Input: part model. Units: mm. Frame: model coordinates. A direction names the side the tool comes from. Coordinates: 2 decimals unless noted, no trailing zeros. Write each loop counter-clockwise with the first axis right and the second up, starting at its lowest first coordinate (ties: lowest second). Pieces come first, ordered by that corner, then holes. Notation, with made-up numbers: (-27.5, -12) - (17.5, -12) arc R35 ccw to (17.5, 22) - close; hole circle Ø4 at (8.25, 70). An arc over 180 degrees is marked (long way). One line per question, with ' | ' between items. Start each with the question number.
1) First-contact query: P1, Ø4, axis at x = -28, z = -2.5, coming from the +Y side; P2, Ø4, axis at x = -7.5, y = -10, coming from the +Z side. Flat tips, straight axial feed; report the tip coordinate or a pass-through.
2) Draft query along X for faces 1 (the flat face through (0, -6, 38.1)), 2 (the flat face through (-38.1, -10, 0)), 3 (the cylindrical face through (-24.984, -6.261, 18.408)). Return one class per face: released by +X, released by -X, zero draft, split by the parting line, or undercut.
3) Section query D-D on x = -28. Return loops of the section in (y, z), and give its area (3 significant figures).
4) Line query: line 1 (X direction, y = -5.5, z = 29.5); line 2 (Z direction, x = -29, y = -5.5); line 3 (Z direction, x = -25, y = -3.25). Output: solid intervals per line, ascending.
5) Section query C-C on y = -2.25. Give the number of separate pieces and of enclosed holes in the cut face, and give its area (3 significant figures).
6) Reachability of faces 4 (the flat face through (-29, -12.7, 29)), 5 (the cylindrical face through (35.927, -6.439, 35.809)), 6 (the flat face through (8, 0, 1)) from +Z, -Z, +X, -X, +Y, -Y: full face, straight path, thin tool, end or side. Return the list, or none.
7) Section query B-B on z = 0. Return loops of the section in (x, y) (3 decimals).
8) Section query A-A on x = 0. Return loops of the section in (y, z) (3 decimals), and give its area (4 significant figures).
```python
from build123d import *

# Parameters (mm, degrees)
F1_DEPTH = 12.7
F3_D     = 11.3284
F4_R     = 7.62
F5_W     = 76.2
F5_H     = 77.0487710834
F6_DEPTH = 7.62
F7_R     = 7.62


# Not quite as in the source:
# - a feature names something its author has since deleted; it is built from what else it names


with BuildPart() as f1:
    # F0 (on Front) → F1 (new body)
    with BuildSketch(Plane.XZ):
        Polygon((-38.1, -38.1), (38.1, -38.1), (38.1, -30.48), (38.1, 38.1), (-38.1, 38.1), align=None)
    extrude(amount=F1_DEPTH)

    # F3 (through all)
    with Locations(Plane.XZ.offset(12.7)):
        with Locations((-29.1592, 29.1592), (-14.5796, 29.1592), (0, 29.1592), (14.5796, 29.1592), (29.1592, 29.1592), (29.1592, 14.5796), (29.1592, 0), (29.1592, -14.5796), (29.1592, -29.1592), (14.5796, -29.1592), (14.5796, -14.5796), (14.5796, 0), (14.5796, 14.5796), (0, 14.5796), (0, 0), (0, -14.5796), (0, -29.1592), (-14.5796, -29.1592), (-14.5796, -14.5796), (-14.5796, 0), (-14.5796, 14.5796), (-29.1592, 14.5796), (-29.1592, 0), (-29.1592, -14.5796), (-29.1592, -29.1592)):
            Hole(F3_D / 2)

    # F4
    f4_edges = [f1.edges().sort_by_distance(p)[0] for p in [
        (-38.1, -6.35, 38.1),
        (38.1, -6.35, 38.1),
        (38.1, -6.35, -38.1),
        (-38.1, -6.35, -38.1),
    ]]
    fillet(f4_edges, radius=F4_R)

    # F5 (on face) → F6 (join)
    with BuildSketch(Plane.XZ.offset(12.7)):
        Rectangle(F5_W, F5_H)
    extrude(amount=F6_DEPTH)

    # F7
    f7_edges = [f1.edges().sort_by_distance(p)[0] for p in [
        (-38.1, -16.51, 38.524386),
        (38.1, -16.51, 38.524386),
        (38.1, -16.51, -38.524386),
        (-38.1, -16.51, -38.524386),
    ]]
    fillet(f7_edges, radius=F7_R)


solid = f1.part
```
Answer key:
1) P1: y = -12.7 | P2: z = 38.1
2) face 1: zero draft | face 2: released by -X | face 3: undercut
3) outline: (-20.32, -38.52) - (-12.7, -38.52) - (-12.7, -38.1) - (0, -38.1) - (0, -34.7) - (-12.7, -34.7) - (-12.7, -23.61) - (0, -23.61) - (0, -20.12) - (-12.7, -20.12) - (-12.7, -9.04) - (0, -9.04) - (0, -5.54) - (-12.7, -5.54) - (-12.7, 5.54) - (0, 5.54) - (0, 9.04) - (-12.7, 9.04) - (-12.7, 20.12) - (0, 20.12) - (0, 23.61) - (-12.7, 23.61) - (-12.7, 34.7) - (0, 34.7) - (0, 38.1) - (-12.7, 38.1) - (-12.7, 38.52) - (-20.32, 38.52) - close | area: 851 mm²
4) line 1: -38.1 to -34.81, -23.51 to -20.23, -8.93 to -5.65, 5.65 to 8.93, 20.23 to 23.51, 34.81 to 38.1 | line 2: -38.1 to -34.82, -23.5 to -20.24, -8.92 to -5.66, 5.66 to 8.92, 20.24 to 23.5, 34.82 to 38.1 | line 3: -38.1 to -33, -25.31 to -18.42, -10.73 to -3.85, 3.85 to 10.73, 18.42 to 25.31, 33 to 38.1
5) separate pieces: 1 | enclosed holes: 25 | area: 3,240 mm²
6) face 4: +Y | face 5: +Z, +X, +Y | face 6: +Z, -Z, +X, -X, +Y
7) outline: (-38.1, -20.32) - (38.1, -20.32) - (38.1, 0) - (34.823, 0) - (34.823, -12.7) - (23.495, -12.7) - (23.495, 0) - (20.244, 0) - (20.244, -12.7) - (8.915, -12.7) - (8.915, 0) - (5.664, 0) - (5.664, -12.7) - (-5.664, -12.7) - (-5.664, 0) - (-8.915, 0) - (-8.915, -12.7) - (-20.244, -12.7) - (-20.244, 0) - (-23.495, 0) - (-23.495, -12.7) - (-34.823, -12.7) - (-34.823, 0) - (-38.1, 0) - close
8) outline: (-20.32, -38.524) - (-12.7, -38.524) - (-12.7, -38.1) - (0, -38.1) - (0, -34.823) - (-12.7, -34.823) - (-12.7, -23.495) - (0, -23.495) - (0, -20.244) - (-12.7, -20.244) - (-12.7, -8.915) - (0, -8.915) - (0, -5.664) - (-12.7, -5.664) - (-12.7, 5.664) - (0, 5.664) - (0, 8.915) - (-12.7, 8.915) - (-12.7, 20.244) - (0, 20.244) - (0, 23.495) - (-12.7, 23.495) - (-12.7, 34.823) - (0, 34.823) - (0, 38.1) - (-12.7, 38.1) - (-12.7, 38.524) - (-20.32, 38.524) - close | area: 835.5 mm²
